from build123d import *

# Parameters (mm, degrees)
ESQUISSE1_W             = 268
ESQUISSE1_H             = 70
BOSS_EXTRU_1_DEPTH      = 6
ESQUISSE2_W             = 50
ESQUISSE2_H             = 6
ESQUISSE2_W_2           = 48
ENL_V_MAT_EXTRU_1_DEPTH = 278.055951028
ESQUISSE3_W             = 6
ESQUISSE3_H             = 20
BOSS_EXTRU_2_DEPTH      = 6
ESQUISSE4_R             = 1.5
ESQUISSE4_W             = 74
ESQUISSE4_H             = 38
ESQUISSE4_W_2           = 3
ESQUISSE4_H_2           = 20
ESQUISSE4_W_3           = 50
ESQUISSE4_H_3           = 30
ENL_V_MAT_EXTRU_2_DEPTH = 10
ESQUISSE5_W             = 6
ESQUISSE5_H             = 19
BOSS_EXTRU_3_DEPTH      = 6
ESQUISSE6_R             = 1.5
ENL_V_MAT_EXTRU_3_DEPTH = 283.863924883
ESQUISSE7_R             = 2.995
ESQUISSE7_R_2           = 3
ENL_V_MAT_EXTRU_4_DEPTH = 3
ESQUISSE8_R             = 1.65
ENL_V_MAT_EXTRU_5_DEPTH = 283.863924883


with BuildPart() as part:
    # Esquisse1 → Boss.-Extru.1 (new body)
    with BuildSketch(Plane.XY):
        with Locations((-134, 35)):
            Rectangle(ESQUISSE1_W, ESQUISSE1_H)
    extrude(amount=BOSS_EXTRU_1_DEPTH)

    # Esquisse2 → Enlèv. mat.-Extru.1 (cut, through all)
    with BuildSketch(Plane.XY.offset(6)):
        with Locations((-243, 3)):
            Rectangle(ESQUISSE2_W, ESQUISSE2_H)
        with Locations((-25, 3)):
            Rectangle(ESQUISSE2_W, ESQUISSE2_H)
        with Locations((-134, 3)):
            Rectangle(ESQUISSE2_W_2, ESQUISSE2_H)
        with Locations((-243, 67)):
            Rectangle(ESQUISSE2_W, ESQUISSE2_H)
        with Locations((-134, 67)):
            Rectangle(ESQUISSE2_W_2, ESQUISSE2_H)
        with Locations((-25, 67)):
            Rectangle(ESQUISSE2_W, ESQUISSE2_H)
    extrude(amount=-ENL_V_MAT_EXTRU_1_DEPTH, mode=Mode.SUBTRACT)

    # Esquisse3 → Boss.-Extru.2 (add)
    with BuildSketch(Plane(origin=(0, 0, 0), x_dir=(0, 0, -1), z_dir=(1, 0, 0))):
        with Locations((-3, 36)):
            Rectangle(ESQUISSE3_W, ESQUISSE3_H)
    extrude(amount=BOSS_EXTRU_2_DEPTH)

    # Esquisse4 → Enlèv. mat.-Extru.2 (cut)
    with BuildSketch(Plane.XY.offset(6)):
        with Locations((-104, 57)):
            Circle(ESQUISSE4_R)
        with Locations((-104, 13)):
            Circle(ESQUISSE4_R)
        with Locations((-10, 57)):
            Circle(ESQUISSE4_R)
        with Locations((-10, 13)):
            Circle(ESQUISSE4_R)
        with Locations((-57, 35)):
            Rectangle(ESQUISSE4_W, ESQUISSE4_H)
        with Locations((-127.5, 35)):
            Rectangle(ESQUISSE4_W_2, ESQUISSE4_H_2)
        with Locations((-208, 43)):
            Rectangle(ESQUISSE4_W_3, ESQUISSE4_H_3)
    extrude(amount=-ENL_V_MAT_EXTRU_2_DEPTH, mode=Mode.SUBTRACT)

    # Esquisse5 → Boss.-Extru.3 (add)
    with BuildSketch(Plane.ZY.offset(268)):
        with Locations((3, 54.5)):
            Rectangle(ESQUISSE5_W, ESQUISSE5_H)
        with Locations((3, 15.5)):
            Rectangle(ESQUISSE5_W, ESQUISSE5_H)
    extrude(amount=BOSS_EXTRU_3_DEPTH)

    # Esquisse6 → Enlèv. mat.-Extru.3 (cut, through all)
    with BuildSketch(Plane(origin=(0, 0, 0), x_dir=(-1, 0, 0), z_dir=(0, 0, -1))):
        with Locations((271, 16)):
            Circle(ESQUISSE6_R)
        with Locations((271, 55)):
            Circle(ESQUISSE6_R)
        with Locations((211, 67)):
            Circle(ESQUISSE6_R)
        with Locations((165, 67)):
            Circle(ESQUISSE6_R)
        with Locations((103, 67)):
            Circle(ESQUISSE6_R)
        with Locations((57, 67)):
            Circle(ESQUISSE6_R)
    extrude(amount=-ENL_V_MAT_EXTRU_3_DEPTH, mode=Mode.SUBTRACT)

    # Esquisse7 → Enlèv. mat.-Extru.4 (cut)
    with BuildSketch(Plane(origin=(0, 0, 0), x_dir=(-1, 0, 0), z_dir=(0, 0, -1))):
        with Locations((271, 16)):
            Circle(ESQUISSE7_R)
        with Locations((271, 55)):
            Circle(ESQUISSE7_R)
        with Locations((211, 67)):
            Circle(ESQUISSE7_R)
        with Locations((165, 67)):
            Circle(ESQUISSE7_R)
        with Locations((103, 67)):
            Circle(ESQUISSE7_R)
        with Locations((57, 67)):
            Circle(ESQUISSE7_R)
        with Locations((104, 57)):
            Circle(ESQUISSE7_R_2)
        with Locations((104, 13)):
            Circle(ESQUISSE7_R_2)
        with Locations((10, 13)):
            Circle(ESQUISSE7_R_2)
        with Locations((10, 57)):
            Circle(ESQUISSE7_R_2)
    extrude(amount=-ENL_V_MAT_EXTRU_4_DEPTH, mode=Mode.SUBTRACT)

    # Esquisse8 → Enlèv. mat.-Extru.5 (cut, through all)
    with BuildSketch(Plane(origin=(0, 0, 0), x_dir=(-1, 0, 0), z_dir=(0, 0, -1))):
        with Locations((116.242255389, 25)):
            Circle(ESQUISSE8_R)
        with Locations((116.242255389, 45)):
            Circle(ESQUISSE8_R)
    extrude(amount=-ENL_V_MAT_EXTRU_5_DEPTH, mode=Mode.SUBTRACT)


solid = part.part
Geometry check sheet. Reference: the model listing, model coordinates, mm. A direction names the side the tool comes from. Round coordinates to 2 decimals unless told otherwise and drop trailing zeros. Order: outer loops, then holes, each group sorted by start corner. A loop starts at its lowest first (then second) coordinate and runs counter-clockwise, first axis right, second up. Notation, with made-up numbers: (62.25, 77.25) - (102.25, 77.25) arc R30 ccw to (102.25, 116.25) - close; hole circle Ø7 at (59.25, 18). An arc over 180 degrees is marked (long way). One line per question, with ' | ' between items. Start each with the question number.
(1) Depth check by flat-ended pin: pin 1 Ø1 at (x, z) = (-145, 4.5) entering from +Y; pin 2 Ø1.8 at (x, z) = (2, 4.5) entering from +Y; pin 3 Ø3.5 at (x, y) = (-165, 67) entering from -Z. Enter the tip coordinate at first touch or a pass-through.
(2) Access from +Z, -Z, +X, -X, +Y, -Y to the whole of each face (thin tool, end or side, straight path). Record for faces 1 (the flat face through (-183, 43, 3)), 2 (the flat face through (-246, 64, 3)), 3 (the flat face through (-272.3, 53.7, 3)).
(3) Sectioned sample at B-B on x = -29. Record the cut outline in (y, z), and give its area (3 significant figures).
(4) Release check for a two-part mould opening along X. For faces 4 (the flat face through (3, 46, 3)), 5 (the cylindrical face through (-273.767, 53.853, 1.479)), 6 (the flat face through (-218, 67, 3)) record: released by +X, released by -X, zero draft, split by the parting line, or undercut.
(5) Thickness scan on L1, parallel to Y at x = -271, z = 0.7 (3 decimals); L2, parallel to X at y = 67, z = 3.95; L3, parallel to Y at x = -10, z = 0.9. Record the ranges inside material, lowest first. Write a range as [from, to].
(6) Sectioned sample at A-A on x = -223. Record the cut outline in (y, z), and give its area (3 significant figures).
Conclusion:
1) pin 1: stops at y = 64 | pin 2: stops at y = 46 | pin 3: stops at z = 3
2) face 1: +Z, -Z | face 2: +Z, -Z, -X, +Y | face 3: -Z
3) outline: (6, 0) - (16, 0) - (16, 6) - (6, 6) - close; (54, 0) - (64, 0) - (64, 6) - (54, 6) - close | area: 120 mm2
4) face 4: zero draft | face 5: undercut | face 6: released by -X
5) L1: y = [6, 13.005], [18.995, 25], [45, 52.005], [57.995, 64] | L2: x = [-218, -212.5], [-209.5, -166.5], [-163.5, -158], [-110, -104.5], [-101.5, -58.5], [-55.5, -50] | L3: y = [6, 10], [16, 54], [60, 64]
6) outline: (6, 0) - (28, 0) - (28, 6) - (6, 6) - close; (58, 0) - (64, 0) - (64, 6) - (58, 6) - close | area: 168 mm2
